Source: CAD feature listing. Evaluate the final solid. Frame: model axes, mm. Give positions to 0.01 mm unless a question says otherwise; leave off trailing zeros. Order: outer loops, then holes, each group sorted by start corner. A loop starts at its lowest first (then second) coordinate and runs counter-clockwise, first axis right, second up. Notation, with made-up numbers: (48, 11) - (58, 11) arc R9 ccw to (58, 23) - close; hole circle Ø5 at (76.25, -7.5). An arc over 180 degrees is marked (long way). Write each question's results on one line, items separated by ' | '. Start each with the question number.
Item 1: Section C-C on x = 2.95. Output: boundary loops of the cut face in (y, z), and give its area (3 significant figures).
Item 2: Mould query, pull axis Z, two halves, no side actions, for faces 1 (the cylindrical face through (3.03, 340.95, 35.82)), 2 (the flat face through (5, 263, 35)). Classes: released by +Z, released by -Z, zero draft, split by the parting line, or undercut.
Item 3: Section B-B on y = 105.5. Output: boundary loops of the cut face in (x, z), and give its area (3 significant figures).
Item 4: Contact query for flat-ended pins moving along their axis: pin 1 Ø1.5 at (x, y) = (3.5, 181) entering from +Z; pin 2 Ø9.5 at (y, z) = (275, 35.03) entering from +X. Output: stop coordinate, or through.
Item 5: Section A-A on y = 275. Output: boundary loops of the cut face in (x, z).
Item 6: Line query: line 1 along Y through (x, z) = (3.1, 31.5); line 2 along Y through (x, z) = (2, 40); line 3 along Z through (x, y) = (3.35, 275). Output: solid intervals per line, ascending.
```python
from build123d import *

# Parameters (mm, degrees)
EXTRUDE_1_DEPTH    = 533.213673317
SKETCH1_R          = 6
CUT_EXTRUDE1_DEPTH = 538.812661937


with BuildPart() as part:
    # Эскиз1 → Вытянуть1 (new body)
    with BuildSketch(Plane(origin=(0, 0, 0), x_dir=(1, 0, 0), z_dir=(0, 1, 0))):
        Polygon((1, 0), (5, 0), (5, -70.068808523), (1, -67.636001514), align=None)
    extrude(amount=EXTRUDE_1_DEPTH)

    # Sketch1 → Cut-Extrude1 (cut, through all)
    with BuildSketch(Plane(origin=(5, 0, 0), x_dir=(0, 0, -1), z_dir=(1, 0, 0))):
        with Locations((-35.034404262, 335)):
            Circle(SKETCH1_R)
        with Locations((-35.034404262, 275)):
            Circle(SKETCH1_R)
    extrude(amount=-CUT_EXTRUDE1_DEPTH, mode=Mode.SUBTRACT)


solid = part.part
```
Evaluation:
1) outline: (0, 0) - (533.21, 0) - (533.21, 68.82) - (0, 68.82) - close; hole circle Ø12 at (275, 35.03); hole circle Ø12 at (335, 35.03) | area: 36,500 mm^2
2) face 1: undercut | face 2: zero draft
3) outline: (1, 0) - (5, 0) - (5, 70.07) - (1, 67.64) - close | area: 275 mm^2
4) pin 1: stops at z = 69.61 | pin 2: passes through
5) outline: (1, 0) - (5, 0) - (5, 29.03) - (1, 29.03) - close; (1, 41.03) - (5, 41.03) - (5, 70.07) - (1, 67.64) - close
6) line 1: y = 0 to 270.15, 279.85 to 330.15, 339.85 to 533.21 | line 2: y = 0 to 271.63, 278.37 to 331.63, 338.37 to 533.21 | line 3: z = 0 to 29.03, 41.03 to 69.07
